Autodesk Inventor part; units mm, degrees
ref_plane "Work Plane1" through (0, 0, 1.5) normal (0, 0, 1) x (1, 0, 0)
ref_plane "YZ Plane" through (0, 0, 0) normal (1, 0, 0) x (0, 1, 0)
ref_plane "XZ Plane" through (0, 0, 0) normal (0, 1, 0) x (-1, 0, 0)
sketch "Sketch1" plane through (0, 0, 0) normal (0, 1, 0) x (-1, 0, 0)
  line L0 (2.25, 2.25) -> (-2.25, 2.25)
  line L1 (-2.25, 2.25) -> (-2.25, -2.25)
  line L2 (-2.25, -2.25) -> (2.25, -2.25)
  line L3 (2.25, -2.25) -> (2.25, 2.25)
  point P0 (0, 0)
  dimension "d0" = 4.5
  dimension "d1" = 2.25
  dimension "d2" = 4.5
  dimension "d3" = 2.25
extrude "Extrusion1" add sketch "Sketch1" along normal blind 3.8
fillet "Fillet1" radius 0.5 4 edges at (2.25, 1.9, 2.25) (2.25, 1.9, -2.25) (-2.25, 1.9, 2.25) (-2.25, 1.9, -2.25)
sketch "Sketch2" plane through (0, 3.8, 0) normal (0, 1, 0) x (1, 0, 0)
  circle A0 centre (0, 0) radius 1.25
  dimension "d7" = 2.5
extrude "Extrusion2" add sketch "Sketch2" along normal blind 3.2
ref_plane "Work Plane1" through (0, 0, 1.5) normal (0, 0, 1) x (1, 0, 0)
sketch "Sketch3" plane through (0, 0, 1.5) normal (0, 0, 1) x (1, 0, 0)
  line L0 (-2.25, 3.8) -> (-2.25, 0)
  line L1 (-2.25, 0.5333) -> (-2.25, 0.2333)
  line L2 (-2.25, 0.2333) -> (-2.3946, 0.2333)
  line L3 (-2.3946, 0.2333) -> (-2.6231, -0.05)
  line L4 (-2.6231, -0.05) -> (-3.25, -0.05)
  line L5 (-3.25, -0.05) -> (-3.25, 0.25)
  line L6 (-3.25, 0.25) -> (-2.8162, 0.25)
  line L7 (-2.8162, 0.25) -> (-2.5878, 0.5333)
  line L8 (-2.5878, 0.5333) -> (-2.25, 0.5333)
  line L9 (-1.75, 0) -> (-2.25, 0)
  point P0 (0, 0)
  dimension "d11" = 0.3
  dimension "d12" = 0.3
  dimension "d13" = 0.05
  dimension "d14" = 1
extrude "Extrusion3" add sketch "Sketch3" along normal mid plane 0.7
mirror "Mirror1" about plane through (0, 0, 0) normal (0, 0, 1) of "Extrusion3"
mirror "Mirror2" about plane through (0, 0, 0) normal (1, 0, 0) of "Extrusion3", "Mirror1"
properties part number "TL3305_Tactile"
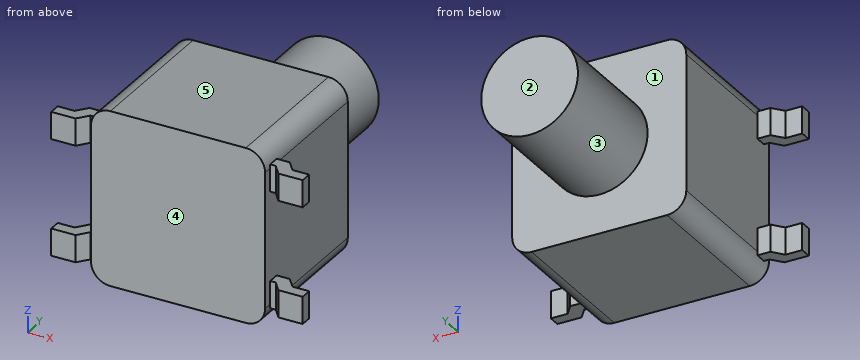
Can you work these out from the model? Positions are in its coordinate system, mm. Face numbers are marked on the shaded views. A direction names the side the tool comes from. Round coordinates to 2 decimals unless told otherwise and drop trailing zeros. Order: outer loops, then holes, each group sorted by start corner. A loop starts at its lowest first (then second) coordinate and runs counter-clockwise, first axis right, second up. Notation, with made-up numbers: (15.25, 74.25) -> (73.25, 74.25) arc R25 ccw to (73.25, 103.25) -> close; hole circle Ø5 at (81.5, 36). An arc over 180 degrees is marked (long way). Return JSON: item names as keys, results as strings. Group by question number.
1. If we section it at D-D, the plane z = -1.5: Write out the boundary of the cut face in (x, y).
2. If we section it at B-B, the plane z = 0: Write out the boundary of the cut face in (x, y).
3. Which directions (+Z, -Z, +X, -X, +Y, -Y) give clear straight access to the entire face, cutting with the end or side of a thin tool? Please do the marked faces 1 and 2.
4. If we section it at A-A, the plane x = 0: Write out the boundary of the cut face in (y, z), then the cut area to 3 significant figures.
5. If we section it at C-C, the plane y = 5: Write out the boundary of the cut face in (x, z).
6. Will these pins go through, and if not, where does the flat tip stop? pin 1 (1.8 mm diameter, centred on y = 2, z = -0.5, fed in from +X); pin 2 (2 mm diameter, centred on x = -1, z = 0, fed in from -Y); pin 3 (1.8 mm diameter, centred on y = 2.5, z = 0.5, fed in from -X).
7. We'd pull the mould along X, two halves only. Please class the marked faces 3, 4 and 5: released by +X, released by -X, zero draft, split by the parting line, or undercut.
8. I need wall thicknesses on line 1 (X direction, y = 3.5, z = 0.2); line 2 (Y direction, x = 0, z = -1); line 3 (Z direction, x = 0, y = 4.5). Which ranges of each line are inside material? Lowest first, please. Write a range as [from, to].
Output values:
{
 "1": {"outline": "(-3.25, -0.05) -> (-2.62, -0.05) -> (-2.39, 0.23) -> (-2.25, 0.23) -> (-2.25, 0) -> (2.25, 0) -> (2.25, 0.23) -> (2.39, 0.23) -> (2.62, -0.05) -> (3.25, -0.05) -> (3.25, 0.25) -> (2.82, 0.25) -> (2.59, 0.53) -> (2.25, 0.53) -> (2.25, 3.8) -> (-2.25, 3.8) -> (-2.25, 0.53) -> (-2.59, 0.53) -> (-2.82, 0.25) -> (-3.25, 0.25) -> close"},
 "2": {"outline": "(-2.25, 0) -> (2.25, 0) -> (2.25, 3.8) -> (1.25, 3.8) -> (1.25, 7) -> (-1.25, 7) -> (-1.25, 3.8) -> (-2.25, 3.8) -> close"},
 "3": {"face 1": "+Y", "face 2": "+Z, -Z, +X, -X, +Y"},
 "4": {"outline": "(0, -2.25) -> (3.8, -2.25) -> (3.8, -1.25) -> (7, -1.25) -> (7, 1.25) -> (3.8, 1.25) -> (3.8, 2.25) -> (0, 2.25) -> close", "area": "25.1 mm²"},
 "5": {"outline": "circle Ø2.5 at (0, 0)"},
 "6": {"pin 1": "x = 2.25", "pin 2": "y = 0", "pin 3": "x = -2.25"},
 "7": {"face 3": "split by the parting line", "face 4": "undercut", "face 5": "zero draft"},
 "8": {"line 1": "[-2.25, 2.25]", "line 2": "[0, 7]", "line 3": "[-1.25, 1.25]"}
}
